Read the model definition and answer for the solid it produces. Units are mm, in the model's axes. Face numbers are marked on the shaded views. A direction names the side the tool comes from. Coordinates: 2 decimals unless noted, no trailing zeros. Order: outer loops, then holes, each group sorted by start corner. A loop starts at its lowest first (then second) coordinate and runs counter-clockwise, first axis right, second up.
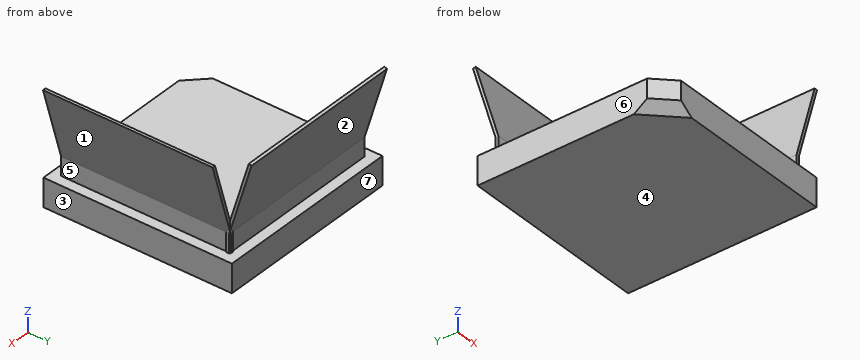
```python
from build123d import *

# Parameters (mm, degrees)
F0_W     = 1000
F0_H     = 150
F1_DEPTH = 500
F3_DEPTH = 450
F5_DEPTH = 450
F6_SIZE  = 100
F7_SIZE  = 50


with BuildPart() as f1:
    # F0 (on Right) → F1 (new body, symmetric)
    with BuildSketch(Plane.YZ):
        Rectangle(F0_W, F0_H)
    extrude(amount=F1_DEPTH, both=True)

    # F2 (on Right) → F3 (join, symmetric)
    with BuildSketch(Plane.YZ):
        Polygon((430, 175), (430, 75), (445, 75), (445, 172.7984674554), (564.1914670014, 570.1033574602), (550, 575), align=None)
    extrude(amount=F3_DEPTH, both=True)

    # F4 (on Front) → F5 (join, symmetric)
    with BuildSketch(Plane.XZ):
        Polygon((430, 175), (430, 75), (445, 75), (445, 172.7984674554), (565.6604597634, 575), (550, 575), align=None)
    extrude(amount=F5_DEPTH, both=True)

    # F6
    f6_edges = [f1.edges().sort_by_distance(p)[0] for p in [
        (-500, -500, 0),
    ]]
    chamfer(f6_edges, length=F6_SIZE)

    # F7
    f7_edges = [f1.edges().sort_by_distance(p)[0] for p in [
        (-450, -450, -75),
    ]]
    chamfer(f7_edges, length=F7_SIZE)


solid = f1.part
```
1) Straight lines are drawn through the part: line 1 (Z direction, x = -87, y = -56); line 2 (Y direction, x = 218.5, z = -15); line 3 (X direction, y = -400.5, z = 104). For each, find the intervals that lie inside material, in ascending order.
A:
line 1: z = -75 to 75
line 2: y = -500 to 500
line 3: x = 430 to 445
2) Determine the mould class of the marked faces 1, 2, 3 and 4 for opening direction Z: pulls with the +Z half, pulls with the -Z half, needs draft (parallel to the pull), parting line crosses it, or undercut.
A:
face 1: undercut
face 2: undercut
face 3: needs draft
face 4: pulls with the -Z half
3) A cutting plane is placed at D-D, the plane z = 99. Determine the outline of the cut face in (x, y), and give its area (3 significant figures).
A:
outline: (-450, 430) - (430, 430) - (430, -450) - (445, -450) - (445, 430) - (450, 430) - (450, 445) - (445, 445) - (445, 450) - (430, 450) - (430, 445) - (-450, 445) - close
area: 26,800 mm2
4) A cutting plane is placed at C-C, the plane z = 485. Determine the outline of the cut face in (x, y).
A:
outline: (-450, 523) - (450, 523) - (450, 538.66) - (-450, 538.66) - close; (523, -450) - (538.66, -450) - (538.66, 450) - (523, 450) - close
5) Which of the six approach directions +Z, -Z, +X, -X, +Y, -Y give full straight-line access (tool end or side, diameter ignored) to the marked faces 5, 6 and 7?
A:
face 5: +X, -Y
face 6: +Z, -Z, -X, +Y, -Y
face 7: -Z, +X, -X, +Y
6) Flat-ended cylindrical pins translate along their axes: pin 1 Ø16 at (y, z) = (441, 149.5) entering from +X; pin 2 Ø1 at (x, y) = (306, 422) entering from +Z; pin 3 Ø5.5 at (x, z) = (448.5, 145.5) entering from -Y. Find the tip coordinate at first contact, or state that the pin passes through.
A:
pin 1: stops at x = 450
pin 2: stops at z = 75
pin 3: stops at y = 430
7) A cutting plane is placed at B-B, the plane y = -61.5. Determine the outline of the cut face in (x, z).
A:
outline: (-500, -75) - (500, -75) - (500, 75) - (445, 75) - (445, 172.8) - (565.66, 575) - (550, 575) - (430, 175) - (430, 75) - (-500, 75) - close
8) A cutting plane is placed at A-A, the plane x = 309. Determine the outline of the cut face in (y, z), and give its area (3 significant figures).
A:
outline: (-500, -75) - (500, -75) - (500, 75) - (445, 75) - (445, 172.8) - (564.19, 570.1) - (550, 575) - (430, 175) - (430, 75) - (-500, 75) - close
area: 158,000 mm2
